Source: CAD feature listing. Evaluate the final solid. Frame: model axes, mm. Face numbers are marked on the shaded views. A direction names the side the tool comes from. Coordinates: 2 decimals unless noted, no trailing zeros. Order: outer loops, then holes, each group sorted by start corner. A loop starts at its lowest first (then second) coordinate and runs counter-clockwise, first axis right, second up. Notation, with made-up numbers: (-7.5, 49.25) -> (29.5, 49.25) arc R26 ccw to (29.5, 73.25) -> close; hole circle Ø1 at (59, 32). An arc over 180 degrees is marked (long way). Put each result on its own line as item: value.
from build123d import *

# Parameters (mm, degrees)
SKETCH1_W           = 76.2
SKETCH1_H           = 25.4
SKETCH1_W_2         = 69.85
SKETCH1_H_2         = 19.05
EXTRUDE_THIN1_DEPTH = 279.4
CUT_EXTRUDE2_DEPTH  = 26.4
SKETCH4_R           = 24.97201
CUT_EXTRUDE3_DEPTH  = 26.4
CUT_EXTRUDE7_DEPTH  = 26.4
SKETCH7_R           = 3.175
CUT_EXTRUDE8_DEPTH  = 77.2
SKETCH8_R           = 3.175
CUT_EXTRUDE9_DEPTH  = 77.2


with BuildPart() as part:
    # Sketch1 → Extrude-Thin1 (new body)
    with BuildSketch(Plane.XY):
        Rectangle(SKETCH1_W, SKETCH1_H)
        Rectangle(SKETCH1_W_2, SKETCH1_H_2, mode=Mode.SUBTRACT)
    extrude(amount=EXTRUDE_THIN1_DEPTH)

    # Sketch3 → Cut-Extrude2 (cut, through all)
    with BuildSketch(Plane(origin=(0, 12.7, 0), x_dir=(1, 0, 0), z_dir=(0, 1, 0))):
        with BuildLine():
            ThreePointArc((-29.73451, -279.4), (-29.157760237, -285.228044516), (-27.449884971, -290.83))
            ThreePointArc((-27.449884971, -290.83), (0, -309.13451), (27.449884971, -290.83))
            ThreePointArc((27.449884971, -290.83), (29.157760237, -285.228044516), (29.73451, -279.4))
            Line((29.73451, -279.4), (-29.73451, -279.4))
        make_face()
        with BuildLine():
            ThreePointArc((29.73451, -279.4), (0, -249.66549), (-29.73451, -279.4))
            Line((-29.73451, -279.4), (29.73451, -279.4))
        make_face()
        with BuildLine():
            ThreePointArc((-29.73451, 0), (-29.157760237, -5.828044516), (-27.449884971, -11.43))
            ThreePointArc((-27.449884971, -11.43), (0, -29.73451), (27.449884971, -11.43))
            ThreePointArc((27.449884971, -11.43), (29.157760237, -5.828044516), (29.73451, 0))
            Line((29.73451, 0), (-29.73451, 0))
        make_face()
        with BuildLine():
            ThreePointArc((29.73451, 0), (0, 29.73451), (-29.73451, 0))
            Line((-29.73451, 0), (29.73451, 0))
        make_face()
    extrude(amount=-CUT_EXTRUDE2_DEPTH, mode=Mode.SUBTRACT)

    # Sketch4 → Cut-Extrude3 (cut, through all)
    with BuildSketch(Plane(origin=(0, 12.7, 0), x_dir=(1, 0, 0), z_dir=(0, 1, 0))):
        with Locations((0, -212.725)):
            Circle(SKETCH4_R)
        with Locations((0, -66.675)):
            Circle(SKETCH4_R)
    extrude(amount=-CUT_EXTRUDE3_DEPTH, mode=Mode.SUBTRACT)

    # Sketch6 → Cut-Extrude7 (cut, through all)
    with BuildSketch(Plane(origin=(0, 12.7, 0), x_dir=(1, 0, 0), z_dir=(0, 1, 0))):
        with BuildLine():
            Line((-38.1, 0), (-38.1, -15.459013065))
            Line((-38.1, -15.459013065), (-25.4, -15.459013065))
            ThreePointArc((-25.4, -15.459013065), (-28.630382803, -8.027594003), (-29.73451, 0))
            Line((-29.73451, 0), (-38.1, 0))
        make_face()
        with BuildLine():
            ThreePointArc((25.4, -15.459013065), (0, -29.73451), (-25.4, -15.459013065))
            Line((-25.4, -15.459013065), (-25.4, -36.257411134))
            ThreePointArc((-25.4, -36.257411134), (-23.662611537, -39.088294047), (-20.351875232, -38.821007943))
            ThreePointArc((-20.351875232, -38.821007943), (0, -32.17799), (20.351875232, -38.821007943))
            ThreePointArc((20.351875232, -38.821007943), (23.662611537, -39.088294047), (25.4, -36.257411134))
            Line((25.4, -36.257411134), (25.4, -15.459013065))
        make_face()
        with BuildLine():
            ThreePointArc((29.73451, 0), (28.630382803, -8.027594003), (25.4, -15.459013065))
            Line((25.4, -15.459013065), (38.1, -15.459013065))
            Line((38.1, -15.459013065), (38.1, 0))
            Line((38.1, 0), (29.73451, 0))
        make_face()
    cut_extrude7 = extrude(amount=-CUT_EXTRUDE7_DEPTH, mode=Mode.SUBTRACT)

    # Sketch7 → Cut-Extrude8 (cut, through all)
    with BuildSketch(Plane(origin=(38.1, 0, 0), x_dir=(0, 0, -1), z_dir=(1, 0, 0))):
        with Locations((-27.686, 0)):
            Circle(SKETCH7_R)
    cut_extrude8 = extrude(amount=-CUT_EXTRUDE8_DEPTH, mode=Mode.SUBTRACT)

    # Mirror3: Cut-Extrude7, Cut-Extrude8 across plane
    add(cut_extrude7.mirror(Plane.XY.offset(139.7)), mode=Mode.SUBTRACT)
    add(cut_extrude8.mirror(Plane.XY.offset(139.7)), mode=Mode.SUBTRACT)

    # Sketch8 → Cut-Extrude9 (cut, through all)
    with BuildSketch(Plane(origin=(38.1, 0, 0), x_dir=(0, 0, -1), z_dir=(1, 0, 0))):
        with Locations((-66.675, 0)):
            Circle(SKETCH8_R)
        with Locations((-212.725, 0)):
            Circle(SKETCH8_R)
    extrude(amount=-CUT_EXTRUDE9_DEPTH, mode=Mode.SUBTRACT)


solid = part.part
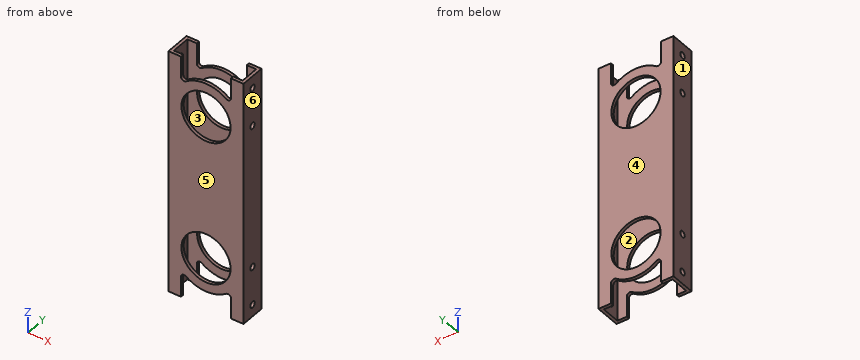
1. Pull-direction query (Y, two-part tool) for the marked faces 3, 4, 5 and 6; classes: pulls with the +Y half, pulls with the -Y half, needs draft (parallel to the pull), parting line crosses it, or undercut.
Numbers:
face 3: undercut
face 4: pulls with the +Y half
face 5: pulls with the -Y half
face 6: needs draft
2. Cut plane C-C on y = -7.25. Output: boundary loops of the cut face in (x, z) (3 decimals), plus the area to 3 significant figures.
Numbers:
outline: (-38.1, 15.459) -> (-34.925, 15.459) -> (-34.925, 263.941) -> (-38.1, 263.941) -> close; (34.925, 15.459) -> (38.1, 15.459) -> (38.1, 263.941) -> (34.925, 263.941) -> close
area: 1,580 mm2
3. First-contact query: pin 1 (5 mm diameter, centred on y = 0, z = 251.714, fed in from +X); pin 2 (8 mm diameter, centred on x = -5.5, y = 10, fed in from +Z). Flat tips, straight axial feed; report the tip coordinate or a pass-through.
Numbers:
pin 1: passes through
pin 2: stops at z = 247.19
4. Set-up query: the marked faces 1 and 2. Return all of +Z, -Z, +X, -X, +Y, -Y with unobstructed straight access to the full face (end or side cutting, diameter ignored); none if empty.
Numbers:
face 1: +Z, -Z, -X, +Y, -Y
face 2: +Z, -Z
5. Cut plane D-D on x = 0. Output: boundary loops of the cut face in (y, z) (3 decimals).
Numbers:
outline: (-12.7, 32.178) -> (-9.525, 32.178) -> (-9.525, 41.703) -> (-12.7, 41.703) -> close; (-12.7, 91.647) -> (-9.525, 91.647) -> (-9.525, 187.753) -> (-12.7, 187.753) -> close; (-12.7, 237.697) -> (-9.525, 237.697) -> (-9.525, 247.222) -> (-12.7, 247.222) -> close; (9.525, 32.178) -> (12.7, 32.178) -> (12.7, 41.703) -> (9.525, 41.703) -> close; (9.525, 91.647) -> (12.7, 91.647) -> (12.7, 187.753) -> (9.525, 187.753) -> close; (9.525, 237.697) -> (12.7, 237.697) -> (12.7, 247.222) -> (9.525, 247.222) -> close
6. Cut plane B-B on z = 133.5. Output: boundary loops of the cut face in (x, y) (3 decimals), plus the area to 3 significant figures.
Numbers:
outline: (-38.1, -12.7) -> (38.1, -12.7) -> (38.1, 12.7) -> (-38.1, 12.7) -> close; hole (-34.925, -9.525) -> (34.925, -9.525) -> (34.925, 9.525) -> (-34.925, 9.525) -> close
area: 605 mm2
7. Ray query, line 1 along Z through (x, y) = (0, 11.15); line 2 along X through (y, z) = (-8.5, 127) (3 decimals); line 3 along Y through (x, z) = (-4, 241) (3 decimals). Return the intervals inside material, ascending.
Numbers:
line 1: z = 32.18 to 41.7, 91.65 to 187.75, 237.7 to 247.22
line 2: x = -38.1 to -34.925, 34.925 to 38.1
line 3: y = -12.7 to -9.525, 9.525 to 12.7
8. Cut plane A-A on x = -32. Output: boundary loops of the cut face in (y, z) (3 decimals), plus the area to 3 significant figures.
Numbers:
outline: (-12.7, 15.459) -> (-9.525, 15.459) -> (-9.525, 263.941) -> (-12.7, 263.941) -> close; (9.525, 15.459) -> (12.7, 15.459) -> (12.7, 263.941) -> (9.525, 263.941) -> close
area: 1,580 mm2
